Here's how the part is built. I have some questions about the finished solid (model axes, mm). A direction names the side the tool comes from. Round coordinates to 2 decimals unless told otherwise and drop trailing zeros. Write each loop counter-clockwise with the first axis right and the second up, starting at its lowest first coordinate (ties: lowest second). Pieces come first, ordered by that corner, then holes. Notation, with made-up numbers: (25, -22) - (49, -22) arc R22 ccw to (49, 4) - close; hole circle Ø3 at (49, 68.25). An arc over 180 degrees is marked (long way). One line per question, with ' | ' between items. Start each with the question number.
(1) Will these pins go through, and if not, where does the flat tip stop? pin 1 (2 mm diameter, centred on x = 1.5, y = 3.5, fed in from +Z); pin 2 (4.5 mm diameter, centred on x = -10.7, y = 10.7, fed in from +Z); pin 3 (2.5 mm diameter, centred on x = 0, y = 0, fed in from +Z); pin 4 (1.2 mm diameter, centred on x = -12.5, y = 1, fed in from -Z).
(2) Imagine slicing it at B-B (y = 0). Write out the boundary of the cut face in (x, z).
(3) Thinking about a two-plate mould opening in Y: for faces 4 (the flat face through (-15, 0, 9)), 5 (the flat face through (-10.286, 3.074, 13.915)), 6 (the flat face through (0, 15, 9)), which applies, pulls with the +Y half, pulls with the -Y half, needs draft (parallel to the pull), parting line crosses it, or undercut?
(4) Imagine slicing it at D-D (z = 12). Write out the boundary of the cut face in (x, y).
(5) Imagine slicing it at C-C (x = 12.25). Write out the boundary of the cut face in (y, z), plus the area to 3 significant figures.
(6) If I drill on L1, parallel to Y at x = -10.7, z = 4.25; L2, parallel to Y at x = 12, z = 3.5; L3, parallel to Y at x = -11.75, z = 7, over which ranges is the centre line in solid material (lowest first)?
(7) Imagine slicing it at A-A (z = 13.75). Write out the boundary of the cut face in (x, y).
(8) For faces 1 (the flat face through (13, 0, 8)), 2 (the flat face through (0, -13, 8)), 3 (the flat face through (3.074, 10.286, 13.915)), which set-ups out of +Z, -Z, +X, -X, +Y, -Y let a thin tool reach every point of the face, with its end or its side?
from build123d import *

# Parameters (mm, degrees)
SKETCH1_W           = 30
SKETCH1_H           = 30
BOSS_EXTRUDE1_DEPTH = 15
CUT_EXTRUDE1_DEPTH  = 15
SKETCH3_R           = 2.5
CUT_EXTRUDE2_DEPTH  = 15
SKETCH4_W           = 7
SKETCH4_H           = 4
BOSS_EXTRUDE2_DEPTH = 30
SKETCH5_W           = 4
SKETCH5_H           = 7
BOSS_EXTRUDE3_DEPTH = 30
CUT_EXTRUDE3_DEPTH  = 2.2
SKETCH7_R           = 1.5
CUT_EXTRUDE4_DEPTH  = 4.5


with BuildPart() as part:
    # Sketch1 → Boss-Extrude1 (new body)
    with BuildSketch(Plane.XY):
        Rectangle(SKETCH1_W, SKETCH1_H)
    extrude(amount=BOSS_EXTRUDE1_DEPTH)

    # Sketch2 → Cut-Extrude1 (cut)
    with BuildSketch(Plane.XY.offset(15)):
        with BuildLine():
            Line((-2, 15), (2, 15))
            Line((2, 15), (2, 10.816653826))
            ThreePointArc((2, 10.816653826), (0, 11), (-2, 10.816653826))
            Line((-2, 10.816653826), (-2, 15))
        make_face()
        with BuildLine():
            Line((15, 2), (15, -2))
            Line((15, -2), (10.816653826, -2))
            ThreePointArc((10.816653826, -2), (11, 0), (10.816653826, 2))
            Line((10.816653826, 2), (15, 2))
        make_face()
        with BuildLine():
            Line((-2, -15), (2, -15))
            Line((2, -15), (2, -10.816653826))
            ThreePointArc((2, -10.816653826), (0, -11), (-2, -10.816653826))
            Line((-2, -10.816653826), (-2, -15))
        make_face()
        with BuildLine():
            Line((-15, -2), (-15, 2))
            Line((-15, 2), (-10.816653826, 2))
            ThreePointArc((-10.816653826, 2), (-11, 0), (-10.816653826, -2))
            Line((-10.816653826, -2), (-15, -2))
        make_face()
    extrude(amount=-CUT_EXTRUDE1_DEPTH, mode=Mode.SUBTRACT)

    # Sketch3 → Cut-Extrude2 (cut)
    with BuildSketch(Plane.XY.offset(15)):
        with Locations((-10.7, 10.7)):
            Circle(SKETCH3_R)
        with Locations((10.7, -10.7)):
            Circle(SKETCH3_R)
    extrude(amount=-CUT_EXTRUDE2_DEPTH, mode=Mode.SUBTRACT)

    # Sketch4 → Boss-Extrude2 (add)
    with BuildSketch(Plane(origin=(15, 0, 0), x_dir=(0, 0, -1), z_dir=(1, 0, 0))):
        with Locations((-11.5, 0)):
            Rectangle(SKETCH4_W, SKETCH4_H)
    extrude(amount=-BOSS_EXTRUDE2_DEPTH)

    # Sketch5 → Boss-Extrude3 (add)
    with BuildSketch(Plane.XZ.offset(15)):
        with Locations((0, 11.5)):
            Rectangle(SKETCH5_W, SKETCH5_H)
    extrude(amount=-BOSS_EXTRUDE3_DEPTH)

    # Sketch6 → Cut-Extrude3 (cut)
    with BuildSketch(Plane.XY.offset(15)):
        with BuildLine():
            Line((-4, 5.437140793), (-2.172951473, 15))
            Line((-2.172951473, 15), (2.172951473, 15))
            Line((2.172951473, 15), (4, 5.437140793))
            ThreePointArc((4, 5.437140793), (4.420928793, 4.420928793), (5.437140793, 4))
            Line((5.437140793, 4), (15, 2.172951473))
            Line((15, 2.172951473), (15, -2.172951473))
            Line((15, -2.172951473), (5.437140793, -4))
            ThreePointArc((5.437140793, -4), (4.420928793, -4.420928793), (4, -5.437140793))
            Line((4, -5.437140793), (2.172951473, -15))
            Line((2.172951473, -15), (-2.172951473, -15))
            Line((-2.172951473, -15), (-4, -5.437140793))
            ThreePointArc((-4, -5.437140793), (-4.420928793, -4.420928793), (-5.437140793, -4))
            Line((-5.437140793, -4), (-15, -2.172951473))
            Line((-15, -2.172951473), (-15, 2.172951473))
            Line((-15, 2.172951473), (-5.437140793, 4))
            ThreePointArc((-5.437140793, 4), (-4.420928793, 4.420928793), (-4, 5.437140793))
        make_face()
    extrude(amount=-CUT_EXTRUDE3_DEPTH, mode=Mode.SUBTRACT)

    # Sketch7 → Cut-Extrude4 (cut)
    with BuildSketch(Plane.XY.offset(15)):
        Circle(SKETCH7_R)
    extrude(amount=-CUT_EXTRUDE4_DEPTH, mode=Mode.SUBTRACT)


solid = part.part
Check sheet entries:
1) pin 1: z = 12.8 | pin 2: through | pin 3: z = 10.5 | pin 4: z = 8
2) outline: (-15, 8) - (-11, 8) - (-11, 0) - (11, 0) - (11, 8) - (15, 8) - (15, 12.8) - (1.5, 12.8) - (1.5, 10.5) - (-1.5, 10.5) - (-1.5, 12.8) - (-15, 12.8) - close
3) face 4: needs draft | face 5: undercut | face 6: pulls with the +Y half
4) outline: (-15, -15) - (15, -15) - (15, 15) - (-15, 15) - close; hole circle Ø5 at (-10.7, 10.7); hole circle Ø3 at (0, 0); hole circle Ø5 at (10.7, -10.7)
5) outline: (-15, 0) - (-12.66, 0) - (-12.66, 15) - (-15, 15) - close; (-8.74, 0) - (-2, 0) - (-2, 8) - (2, 8) - (2, 0) - (15, 0) - (15, 15) - (2.7, 15) - (2.7, 12.8) - (-2.7, 12.8) - (-2.7, 15) - (-8.74, 15) - close | area: 347 mm^2
6) L1: -15 to 8.2, 13.2 to 15 | L2: -15 to -12.84, -8.56 to -2, 2 to 15 | L3: -15 to -2, 2 to 8.43, 12.97 to 15
7) outline: (-15, -15) - (-2.17, -15) - (-4, -5.44) arc R1.44 ccw to (-5.44, -4) - (-15, -2.17) - close; (-15, 2.17) - (-5.44, 4) arc R1.44 ccw to (-4, 5.44) - (-2.17, 15) - (-15, 15) - close; (2.17, -15) - (15, -15) - (15, -2.17) - (5.44, -4) arc R1.44 ccw to (4, -5.44) - close; (2.17, 15) - (4, 5.44) arc R1.44 ccw to (5.44, 4) - (15, 2.17) - (15, 15) - close; hole circle Ø5 at (-10.7, 10.7); hole circle Ø5 at (10.7, -10.7)
8) face 1: -Z, +X | face 2: -Z, -Y | face 3: +Z
